Autodesk Inventor part; units mm, degrees
ref_plane "1_XY" through (0, 0, 0) normal (0, 1, 0) x (1, 0, 0)
ref_plane "1_YZ" through (0, 0, 0) normal (1, 0, 0) x (0, 0, -1)
ref_plane "1_ZX" through (0, 0, 0) normal (0, 0, -1) x (0, 1, 0)
sketch "Sketch_1" plane through (0, 0, 0) normal (0, 1, 0) x (-1, 0, 0)
  line L0 (8.382, -3.558) -> (8.382, 3.558)
  arc A0 (8.382, 3.558) -> (8.382, -3.558) centre (0, 0) ccw
  arc A1 (5.0033, 1.016) -> (5.0033, -1.016) centre (0, 0) ccw
  line L1 (5.0033, -1.016) -> (4.3053, -1.016)
  line L2 (4.3053, -1.016) -> (4.3053, 1.016)
  line L3 (4.3053, 1.016) -> (5.0033, 1.016)
extrude "Extrusion1" add sketch "Sketch_1" along normal mid plane 0.9906
sketch "Sketch_2" plane through (0, 0, 0) normal (0, 0, 1) x (1, 0, 0)
  arc A0 (-9.1059, 0.2667) -> (-8.3439, -0.4953) centre (-8.3439, 0.2667) ccw
  line L0 (-8.3439, -0.4953) -> (-8.1153, -0.4953)
  line L1 (-8.1153, -0.4953) -> (-8.1153, 2.2987)
  line L2 (-8.1153, 2.2987) -> (-9.1059, 2.2987)
  line L3 (-9.1059, 2.2987) -> (-9.1059, 0.2667)
extrude "Extrusion2" add sketch "Sketch_2" along normal mid plane 2.794
ref_plane "1_XY" through (0, 0, 0) normal (0, 1, 0) x (1, 0, 0)
ref_plane "1_YZ" through (0, 0, 0) normal (1, 0, 0) x (0, 0, -1)
ref_plane "1_ZX" through (0, 0, 0) normal (0, 0, -1) x (0, 1, 0)
properties part number "AT518"
Check sheet for the modelled part. Datum: model origin and axes. Units: mm. A direction names the side the tool comes from. Round coordinates to 2 decimals unless told otherwise and drop trailing zeros. Order: outer loops, then holes, each group sorted by start corner. A loop starts at its lowest first (then second) coordinate and runs counter-clockwise, first axis right, second up.
(1) Cross-section at B-B, the plane x = 0. Enter the section's corners in (y, z), and give its area (3 significant figures).
(2) Access from +Z, -Z, +X, -X, +Y, -Y to the whole of each face (thin tool, end or side, straight path). Record for faces 4 (the flat face through (-8.6, 2.299, 0)), 5 (the flat face through (-8.115, 1, 0)).
(3) Cross-section at C-C, the plane y = 2. Enter the section's corners in (x, z), and give its area (3 significant figures).
(4) Draft check along X on faces 1 (the cylindrical face through (9.1, 0, -0.3)), 2 (the flat face through (-9.106, 1, 0)), 3 (the flat face through (-4.305, 0, 0)). Enter one of: pulls with the +X half, pulls with the -X half, needs draft (parallel to the pull), parting line crosses it, or undercut.
(5) Cross-section at D-D, the plane z = 2.25. Enter the section's corners in (x, y), and give its area (3 significant figures).
(6) Scan lines: probe 1 along Z at (x, y) = (0, -0.1); probe 2 along X at (y, z) = (0.2, 0); probe 3 along Y at (x, z) = (-5.5, 4). Record each from-to range of solid material in increasing order.
(7) Go/stop test with flat-tipped pins: P1, Ø6, axis at x = 0, z = 0, coming from the -Y side; P2, Ø6, axis at x = 0, z = 3, coming from the +Y side; P3, Ø0.6, axis at x = -4.5, y = 0, coming from the +Z side; P4, Ø0.5, axis at y = 1.5, z = 0, coming from the +X side. Record where each tip stops, or that it passes through.
Check sheet entries:
1. outline: (-0.5, -9.11) - (0.5, -9.11) - (0.5, -5.11) - (-0.5, -5.11) - close; (-0.5, 5.11) - (0.5, 5.11) - (0.5, 9.11) - (-0.5, 9.11) - close
1. area: 7.93 mm2
2. face 4: +Z, -Z, +X, -X, +Y
2. face 5: +Z, -Z, +X, +Y
3. outline: (-9.11, -1.4) - (-8.12, -1.4) - (-8.12, 1.4) - (-9.11, 1.4) - close
3. area: 2.77 mm2
4. face 1: parting line crosses it
4. face 2: pulls with the -X half
4. face 3: undercut
5. outline: (-8.38, -0.5) - (-4.58, -0.5) - (-4.58, 0.5) - (-8.38, 0.5) - close; (4.58, -0.5) - (8.82, -0.5) - (8.82, 0.5) - (4.58, 0.5) - close
5. area: 7.96 mm2
6. probe 1: z = -9.11 to -5.11, 5.11 to 9.11
6. probe 2: x = -9.1 to -4.31, 5.11 to 9.11
6. probe 3: y = -0.5 to 0.5
7. P1: passes through
7. P2: stops at y = 0.5
7. P3: stops at z = 8.08
7. P4: stops at x = -8.12
